from build123d import *

# Parameters (mm, degrees)
BOSS_EXTRUDE1_DEPTH = 12.7
SKETCH14_R          = 4
SKETCH14_R_2        = 1.63195
CUT_EXTRUDE1_DEPTH  = 12.7
SKETCH14_3_R        = 1.63195
CUT_EXTRUDE2_DEPTH  = 158.035218157
CUT_EXTRUDE3_DEPTH  = 169.185284783
FILLET1_R           = 5
FILLET2_R           = 1
SKETCH16_R          = 4.7625
CUT_EXTRUDE4_DEPTH  = 169.185284738


with BuildPart() as part:
    # Sketch1 → Boss-Extrude1 (new body)
    with BuildSketch(Plane.XY):
        with BuildLine():
            Line((0, -150), (0, -114.3))
            ThreePointArc((0, -114.3), (-40.036431777, -107.058741495), (-75, -86.252478225))
            Line((-75, -86.252478225), (-75, -150))
            Line((-75, -150), (0, -150))
        make_face()
        with BuildLine():
            ThreePointArc((75, -86.252478225), (40.036431777, -107.058741495), (0, -114.3))
            Line((0, -114.3), (0, -150))
            Line((0, -150), (75, -150))
            Line((75, -150), (75, -86.252478225))
        make_face()
    extrude(amount=BOSS_EXTRUDE1_DEPTH)

    # Sketch14 → Cut-Extrude1 (cut, symmetric)
    # profile 1 of 2: a face of its own
    with BuildSketch(Plane(origin=(-75.884162529, -108.373815459, 0), x_dir=(-0.8191520442889954, 0.5735764363510409, 0), z_dir=(0.5735764363510409, 0.8191520442889954, 0))):
        with Locations((0, 6.35)):
            Circle(SKETCH14_R)
        with Locations((0, 6.35)):
            Circle(SKETCH14_R_2, mode=Mode.SUBTRACT)
    # profile 2 of 2: a face of its own
    with BuildSketch(Plane(origin=(-75.884162529, -108.373815459, 0), x_dir=(-0.8191520442889954, 0.5735764363510409, 0), z_dir=(0.5735764363510409, 0.8191520442889954, 0))):
        with Locations((0, 6.35)):
            Circle(SKETCH14_R_2)
    cut_extrude1 = extrude(amount=CUT_EXTRUDE1_DEPTH, both=True, mode=Mode.SUBTRACT)

    # Sketch14_3 → Cut-Extrude2 (cut, through all)
    with BuildSketch(Plane(origin=(-75.884162529, -108.373815459, 0), x_dir=(-0.8191520442889954, 0.5735764363510409, 0), z_dir=(0.5735764363510409, 0.8191520442889954, 0))):
        with Locations(Location((0, 6.35, 0), (0, 0, 180))):
            Circle(SKETCH14_3_R)
    cut_extrude2 = extrude(amount=CUT_EXTRUDE2_DEPTH, mode=Mode.SUBTRACT)

    # Mirror1: Cut-Extrude1, Cut-Extrude2 across plane
    add(cut_extrude1.mirror(Plane(origin=(0, 0, 0), x_dir=(0, 0, 1), z_dir=(1, 0, 0))), mode=Mode.SUBTRACT)
    add(cut_extrude2.mirror(Plane(origin=(0, 0, 0), x_dir=(0, 0, 1), z_dir=(1, 0, 0))), mode=Mode.SUBTRACT)

    # Sketch15 → Cut-Extrude3 (cut, through all)
    with BuildSketch(Plane.XY.offset(12.7)):
        Polygon((0, -150), (0, -130), (-48.452994616, -130), (-60, -150), align=None)
        Polygon((48.452994616, -130), (0, -130), (0, -150), (60, -150), align=None)
    extrude(amount=-CUT_EXTRUDE3_DEPTH, mode=Mode.SUBTRACT)

    # Fillet1
    fillet1_edges = [part.edges().sort_by_distance(p)[0] for p in [
        (60, -150, 6.35),
        (-60, -150, 6.35),
        (-48.452994616, -130, 6.35),
        (48.452994616, -130, 6.35),
        (-75, -86.252478225, 6.35),
        (75, -86.252478225, 6.35),
    ]]
    fillet(fillet1_edges, radius=FILLET1_R)

    # Fillet2
    fillet2_edges = [part.edges().sort_by_distance(p)[0] for p in [
        (-75, -123.302406772, 12.7),
        (-68.943375673, -150, 12.7),
        (-75, -123.302406772, 0),
        (75, -123.302406772, 0),
        (0, -114.3, 0),
        (0, -114.3, 12.7),
        (-68.943375673, -150, 0),
        (-54.226497308, -140, 0),
        (68.943375673, -150, 0),
        (54.226497308, -140, 0),
        (0, -130, 0),
        (-72.272784424, -92.151224996, 0),
        (-60.386751346, -149.330127019, 0),
        (60.386751346, -149.330127019, 0),
        (72.272784424, -92.151224996, 0),
        (-54.226497308, -140, 12.7),
        (0, -130, 12.7),
        (54.226497308, -140, 12.7),
        (68.943375673, -150, 12.7),
        (-72.272784424, -92.151224996, 12.7),
        (-60.386751346, -149.330127019, 12.7),
        (60.386751346, -149.330127019, 12.7),
        (72.272784424, -92.151224996, 12.7),
        (48.06624327, -130.669872981, 12.7),
        (48.06624327, -130.669872981, 0),
        (-75, -150, 6.35),
        (-48.06624327, -130.669872981, 12.7),
        (-48.06624327, -130.669872981, 0),
        (75, -123.302406772, 12.7),
        (75, -150, 6.35),
    ]]
    fillet(fillet2_edges, radius=FILLET2_R)

    # Sketch16 → Cut-Extrude4 (cut, through all)
    with BuildSketch(Plane.XY.offset(12.7)):
        with Locations((-55.95, -116.345)):
            Circle(SKETCH16_R)
        with Locations(Location((55.95, -116.345, 0), (0, 0, 180))):
            Circle(SKETCH16_R)
    extrude(amount=-CUT_EXTRUDE4_DEPTH, mode=Mode.SUBTRACT)


solid = part.part
For this review, take the finished solid that the model builds, in its own axes (mm). A direction names the side the tool comes from. Give positions to 0.01 mm unless a question says otherwise; leave off trailing zeros.
Item 1: Insertion check: pin 1 (3 mm diameter, centred on x = 10, z = 7.5, fed in from +Y). The pin has a flat end and moves straight along its axis. Give the tip position at first contact, or say it passes through.
Item 2: For line 1 along X through (y, z) = (-114.5, 6.5); line 2 along X through (y, z) = (-134, 10.5); line 3 along X through (y, z) = (-100, 5), list the stretches that pass through material, from the lowest coordinate up.
Item 3: Tool access review of faces 5 (the cylindrical face through (54.548, -139.955, 12.415)), 6 (the flat face through (-70.01, -96.983, 5.517)), 7 (the cylindrical face through (60.42, -149.35, 6.28)), 8 (the flat face through (-1, -120, 0)), 9 (the cylindrical face through (54.548, -139.955, 0.285)): name each direction out of +Z, -Z, +X, -X, +Y, -Y from which nothing blocks a thin tool from reaching the whole face with its end or side.
Item 4: Draft analysis for pull direction X (two halves, no side actions). For faces 1 (the flat face through (-75, -122, 6)), 2 (the cylindrical face through (72.204, -92.117, 6.425)), 3 (the cylindrical face through (-69.07, -105.61, 6.53)), 4 (the flat face through (68, -150, 6)), state which applies: +X half, -X half, draft (parallel to the pull), parting line (faces both ways), or undercut.
Calculated:
1. pin 1: stops at y = -113.72
2. line 1: x = -75 to -60.34, -51.56 to 51.56, 60.34 to 75
2. line 2: x = -75 to -50.76, 50.76 to 75
2. line 3: x = -75 to -74.62, -65.7 to -55.36, 55.36 to 65.7, 74.62 to 75
3. face 5: +Z, -Y
3. face 6: none
3. face 7: +Z, -Z, -Y
3. face 8: -Z, +X, -X, +Y, -Y
3. face 9: -Z, -Y
4. face 1: -X half
4. face 2: undercut
4. face 3: undercut
4. face 4: draft
